Check sheet for the modelled part. Datum: model origin and axes. Units: mm. Face numbers are marked on the shaded views. A direction names the side the tool comes from. Coordinates: 2 decimals unless noted, no trailing zeros. Write each loop counter-clockwise with the first axis right and the second up, starting at its lowest first coordinate (ties: lowest second). Pieces come first, ordered by that corner, then holes. Notation, with made-up numbers: (13, 9.5) -> (67, 9.5) arc R17 cw to (67, 21.5) -> close; hole circle Ø10 at (82.25, 80). An arc over 180 degrees is marked (long way). One line per item, written item: value. Start each with the question number.
1) Set-up check for the marked faces 4, 5 and 6: record each of +Z, -Z, +X, -X, +Y, -Y from which the full face is reachable in a straight line by a thin tool's end or side.
2) Draft check along X on the marked faces 1, 2 and 3. Enter one of: +X half, -X half, draft (parallel to the pull), parting line (faces both ways), or undercut.
3) Sectioned sample at A-A on x = 0. Enter the section's corners in (y, z).
4) Sectioned sample at B-B on y = 1.75. Give the number of separate pieces and of enclosed holes in the cut face, plus the area to 3 significant figures.
5) Sectioned sample at D-D on x = -6. Enter the section's corners in (y, z), plus the area to 3 significant figures.
6) Gauge pin test, flat ends, axial feed: P1, Ø3, axis at y = 2.5, z = 5, coming from the +X side; P2, Ø1, axis at x = -8, y = 2, coming from the +Z side; P3, Ø5, axis at x = -9, z = 9.5, coming from the +Y side. Record the tip position at first contact, or that the pin passes through.
7) Scan lines: line 1 along X through (y, z) = (2.75, 11.5); line 2 along X through (y, z) = (3, 9.5); line 3 along Z through (x, y) = (-6, 4). Record each from-to range of solid material in increasing order. Write a range as [from, to].
8) Sectioned sample at C-C on z = -10. Enter the section's corners in (x, y), plus the area to 3 significant figures.
```python
from build123d import *
from build123d.topology import SkipClean

# Parameters (mm, degrees)
SKETCH_1_R          = 15
EXTRUDE_1_DEPTH     = 6.6
EXTRUDE_2_DEPTH     = 2
SKETCH_3_R          = 17
SKETCH_3_R_2        = 15
EXTRUDE_3_DEPTH     = 5.3
SKETCH_4_R          = 17
SKETCH_4_R_2        = 15
CUT_EXTRUDE_3_DEPTH = 1.3


with BuildPart() as part:
    # 草图1 → 凸台-拉伸1 (new body)
    with BuildSketch(Plane(origin=(0, 0, 0), x_dir=(1, 0, 0), z_dir=(0, 1, 0))):
        with Locations(Location((0, 0, 0), (0, 0, 270))):
            Circle(SKETCH_1_R)
        with BuildLine():
            Line((1.118033989, -1), (-1.118033989, -1))
            ThreePointArc((-1.118033989, -1), (-1.4531398, 0.37200097), (-0.5, 1.414213562))
            Line((-0.5, 1.414213562), (-0.5, 3.464101615))
            ThreePointArc((-0.5, 3.464101615), (-0.874472135, 3.388996678), (-1.23853126, 3.273536363))
            ThreePointArc((-1.23853126, 3.273536363), (-2.407810688, 3.08721539), (-3.555224024, 3.379401158))
            Line((-3.555224024, 3.379401158), (-8.04299568, 6.641703286))
            ThreePointArc((-8.04299568, 6.641703286), (-8.733606232, 8.638127636), (-7.69519148, 10.477787366))
            ThreePointArc((-7.69519148, 10.477787366), (0, 13), (7.69519148, 10.477787366))
            ThreePointArc((7.69519148, 10.477787366), (8.733606232, 8.638127636), (8.04299568, 6.641703286))
            Line((8.04299568, 6.641703286), (3.555224024, 3.379401158))
            ThreePointArc((3.555224024, 3.379401158), (2.407810688, 3.08721539), (1.23853126, 3.273536363))
            ThreePointArc((1.23853126, 3.273536363), (0.874472135, 3.388996678), (0.5, 3.464101615))
            Line((0.5, 3.464101615), (0.5, 1.414213562))
            ThreePointArc((0.5, 1.414213562), (1.4531398, 0.37200097), (1.118033989, -1))
        make_face(mode=Mode.SUBTRACT)
        with BuildLine():
            Line((-1.149035241, -4.7686149), (-1.73038593, -10.286290225))
            ThreePointArc((-1.73038593, -10.286290225), (-3.114034858, -11.882588681), (-5.226434294, -11.903124992))
            ThreePointArc((-5.226434294, -11.903124992), (-11.258330249, -6.5), (-12.921625774, 1.425337626))
            ThreePointArc((-12.921625774, 1.425337626), (-11.847641089, 3.244461045), (-9.77338161, 3.644586939))
            Line((-9.77338161, 3.644586939), (-4.704259264, 1.389213742))
            ThreePointArc((-4.704259264, 1.389213742), (-3.877512299, 0.541617529), (-3.45423128, -0.564168647))
            ThreePointArc((-3.45423128, -0.564168647), (-3.031088913, -1.75), (-2.21570002, -2.709367716))
            ThreePointArc((-2.21570002, -2.709367716), (-1.469701611, -3.628832918), (-1.149035241, -4.7686149))
        make_face(mode=Mode.SUBTRACT)
        with BuildLine():
            Line((1.149035241, -4.7686149), (1.73038593, -10.286290225))
            ThreePointArc((1.73038593, -10.286290225), (3.114034858, -11.882588681), (5.226434294, -11.903124992))
            ThreePointArc((5.226434294, -11.903124992), (11.258330249, -6.5), (12.921625774, 1.425337626))
            ThreePointArc((12.921625774, 1.425337626), (11.847641089, 3.244461045), (9.77338161, 3.644586939))
            Line((9.77338161, 3.644586939), (4.704259264, 1.389213742))
            ThreePointArc((4.704259264, 1.389213742), (3.877512299, 0.541617529), (3.45423128, -0.564168647))
            ThreePointArc((3.45423128, -0.564168647), (3.031088913, -1.75), (2.21570002, -2.709367716))
            ThreePointArc((2.21570002, -2.709367716), (1.469701611, -3.628832918), (1.149035241, -4.7686149))
        make_face(mode=Mode.SUBTRACT)
    extrude(amount=EXTRUDE_1_DEPTH)

    # 草图2 → 凸台-拉伸2 (add)
    with BuildSketch(Plane(origin=(0, 6.6, 0), x_dir=(1, 0, 0), z_dir=(0, 1, 0))):
        with BuildLine():
            ThreePointArc((3.45423128, -0.564168647), (3.488539055, -0.283011059), (3.5, 0))
            ThreePointArc((3.5, 0), (2.879657915, 1.989364294), (1.23853126, 3.273536363))
            ThreePointArc((1.23853126, 3.273536363), (0.874472135, 3.388996678), (0.5, 3.464101615))
            Line((0.5, 3.464101615), (0.5, 1.414213562))
            ThreePointArc((0.5, 1.414213562), (1.4531398, 0.37200097), (1.118033989, -1))
            Line((1.118033989, -1), (-1.118033989, -1))
            ThreePointArc((-1.118033989, -1), (-1.4531398, 0.37200097), (-0.5, 1.414213562))
            Line((-0.5, 1.414213562), (-0.5, 3.464101615))
            ThreePointArc((-0.5, 3.464101615), (-0.874472135, 3.388996678), (-1.23853126, 3.273536363))
            ThreePointArc((-1.23853126, 3.273536363), (-3.031088913, 1.75), (-3.45423128, -0.564168647))
            ThreePointArc((-3.45423128, -0.564168647), (-3.031088913, -1.75), (-2.21570002, -2.709367716))
            ThreePointArc((-2.21570002, -2.709367716), (0, -3.5), (2.21570002, -2.709367716))
            ThreePointArc((2.21570002, -2.709367716), (3.031088913, -1.75), (3.45423128, -0.564168647))
        make_face()
    extrude(amount=EXTRUDE_2_DEPTH)

    # 倒角1: read off the stored shape, not the designer's step
    # 倒角1 outline → 倒角1 (revolve, cut)
    with BuildSketch(Plane.XY):
        Polygon((3.5, 8.6), (2.5, 8.6), (3.5, 7.6), align=None)
    revolve(axis=Axis((0, 0, 0), (0, 1, 0)), mode=Mode.SUBTRACT)

    # 草图3 → 凸台-拉伸3 (add)
    with SkipClean():  # the faces are left unmerged after this step: merging them gives an invalid solid
        with BuildSketch(Plane(origin=(0, 0, 0), x_dir=(1, 0, 0), z_dir=(0, 1, 0))):
            with Locations(Location((0, 0, 0), (0, 0, 270))):
                Circle(SKETCH_3_R)
            with Locations(Location((0, 0, 0), (0, 0, 270))):
                Circle(SKETCH_3_R_2, mode=Mode.SUBTRACT)
        extrude(amount=EXTRUDE_3_DEPTH)

    # 草图4 → 切除-拉伸3 (cut)
    with SkipClean():  # the faces are left unmerged after this step: merging them gives an invalid solid
        with BuildSketch(Plane.XZ):
            with Locations(Location((0, 0, 0), (0, 0, 270))):
                Circle(SKETCH_4_R)
            with Locations(Location((0, 0, 0), (0, 0, 90))):
                Circle(SKETCH_4_R_2, mode=Mode.SUBTRACT)
        extrude(amount=-CUT_EXTRUDE_3_DEPTH, mode=Mode.SUBTRACT)


solid = part.part
```
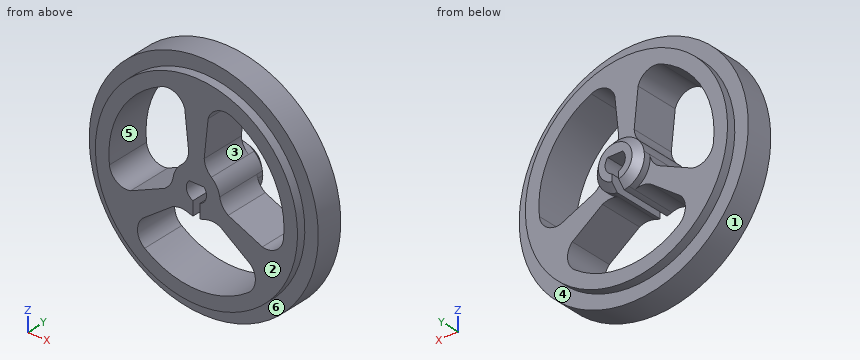
Answers:
1. face 4: +Y
1. face 5: +Y, -Y
1. face 6: -Y
2. face 1: parting line
2. face 2: draft
2. face 3: undercut
3. outline: (0, -15) -> (1.3, -15) -> (1.3, -17) -> (5.3, -17) -> (5.3, -15) -> (6.6, -15) -> (6.6, -13) -> (0, -13) -> close; (0, 1) -> (8.6, 1) -> (8.6, 2.5) -> (7.6, 3.5) -> (6.6, 3.5) -> (6.6, 15) -> (5.3, 15) -> (5.3, 17) -> (1.3, 17) -> (1.3, 15) -> (0, 15) -> close
4. separate pieces: 1
4. enclosed holes: 3
4. area: 509 mm2
5. outline: (0, -13.75) -> (1.3, -13.75) -> (1.3, -15.91) -> (5.3, -15.91) -> (5.3, -13.75) -> (6.6, -13.75) -> (6.6, -11.53) -> (0, -11.53) -> close; (0, -5.16) -> (6.6, -5.16) -> (6.6, -1.97) -> (0, -1.97) -> close; (0, 11.53) -> (6.6, 11.53) -> (6.6, 13.75) -> (5.3, 13.75) -> (5.3, 15.91) -> (1.3, 15.91) -> (1.3, 13.75) -> (0, 13.75) -> close
5. area: 67.6 mm2
6. P1: stops at x = 16.64
6. P2: stops at z = 15.26
6. P3: stops at y = 6.6
7. line 1: x = [-12.52, -6.06], [-2.52, 2.52], [6.06, 12.52]
7. line 2: x = [-14.1, -8.87], [-1.65, 1.65], [8.87, 14.1]
7. line 3: z = [-15.91, -11.53], [-5.16, -1.97], [11.53, 15.91]
8. outline: (-13.75, 1.3) -> (-11.18, 1.3) -> (-11.18, 0) -> (-8.19, 0) -> (-8.19, 6.6) -> (-11.18, 6.6) -> (-11.18, 5.3) -> (-13.75, 5.3) -> close; (8.19, 0) -> (11.18, 0) -> (11.18, 1.3) -> (13.75, 1.3) -> (13.75, 5.3) -> (11.18, 5.3) -> (11.18, 6.6) -> (8.19, 6.6) -> close
8. area: 60.0 mm2
